```python
from build123d import *

# Parameters (mm, degrees)
SKETCH_1_W                         = 12
SKETCH_1_H                         = 8
EXTRUDE_1_DEPTH                    = 350
CUT_EXTRUDE_1_DEPTH                = 351
CHAMFER_1_SIZE                     = 0.5
PATTERN_LINEAR_1_COUNT             = 9
PATTERN_LINEAR_1_PITCH             = 40
CHAMFER_1_OF_PATTERN_LINEAR_1_SIZE = 0.5
CHAMFER_2_SIZE                     = 0.3


with BuildPart() as part:
    # Эскиз1 → Бобышка-Вытянуть1 (new body)
    with BuildSketch(Plane(origin=(0, 0, 0), x_dir=(1, 0, 0), z_dir=(0, 1, 0))):
        with Locations((6, 4)):
            Rectangle(SKETCH_1_W, SKETCH_1_H)
    extrude(amount=EXTRUDE_1_DEPTH)

    # Эскиз2 → Вырез-Вытянуть1 (cut, through all)
    with BuildSketch(Plane(origin=(0, 350, 0), x_dir=(1, 0, 0), z_dir=(0, 1, 0))):
        with BuildLine():
            Line((11, 2.25), (11, 1.75))
            Line((11, 1.75), (11.5, 1.75))
            ThreePointArc((11.5, 1.75), (11.706107374, 1.524471742), (12, 1.440983006))
            Line((12, 1.440983006), (12, 2.559016994))
            ThreePointArc((12, 2.559016994), (11.706107374, 2.475528258), (11.5, 2.25))
            Line((11.5, 2.25), (11, 2.25))
        make_face()
    cut_extrude_1 = extrude(amount=-CUT_EXTRUDE_1_DEPTH, mode=Mode.SUBTRACT)

    # Зеркальное отражение1: Вырез-Вытянуть1 across plane
    add(cut_extrude_1.mirror(Plane(origin=(6, 0, 0), x_dir=(0, 0, 1), z_dir=(1, 0, 0))), mode=Mode.SUBTRACT)

    # Эскиз4 → Вырез-Повернуть1 (revolve, cut)
    with BuildSketch(Plane(origin=(6, 0, 0), x_dir=(0, 0, -1), z_dir=(1, 0, 0))):
        Polygon((0, 339), (4.5, 339), (4.5, 337.25), (8, 337.25), (8, 335), (0, 335), align=None)
    cut_revolve_1 = revolve(axis=Axis((6, 335, -8), (0, 0, 1)), mode=Mode.SUBTRACT)

    # Фаска1
    chamfer_1_edges = [part.edges().sort_by_distance(p)[0] for p in [
        (6, 331, 0),
        (6, 332.75, -8),
    ]]
    chamfer(chamfer_1_edges, length=CHAMFER_1_SIZE)

    # Линейный массив1: Вырез-Повернуть1 ×9
    with Locations(*[(0, -i * PATTERN_LINEAR_1_PITCH, 0) for i in range(1, PATTERN_LINEAR_1_COUNT)]):
        add(cut_revolve_1, mode=Mode.SUBTRACT)

    # Фаска1 of Линейный массив1
    chamfer_1_of_pattern_linear_1_edges = [part.edges().sort_by_distance(p)[0] for p in [
        (6, 291, 0),
        (6, 292.75, -8),
        (6, 251, 0),
        (6, 252.75, -8),
        (6, 211, 0),
        (6, 212.75, -8),
        (6, 171, 0),
        (6, 172.75, -8),
        (6, 131, 0),
        (6, 132.75, -8),
        (6, 91, 0),
        (6, 92.75, -8),
        (6, 51, 0),
        (6, 52.75, -8),
        (6, 11, 0),
        (6, 12.75, -8),
    ]]
    chamfer(chamfer_1_of_pattern_linear_1_edges, length=CHAMFER_1_OF_PATTERN_LINEAR_1_SIZE)

    # Фаска2
    chamfer_2_edges = [part.edges().sort_by_distance(p)[0] for p in [
        (12, 350, -0.720491503),
        (6, 350, -8),
        (12, 0, -5.279508497),
        (12, 350, -5.279508497),
        (11.25, 0, -2.25),
        (11.706107374, 0, -2.475528258),
        (11.706107374, 0, -1.524471742),
        (11.25, 0, -1.75),
        (11, 0, -2),
        (11.25, 350, -2.25),
        (11, 350, -2),
        (11.25, 350, -1.75),
        (11.706107374, 350, -1.524471742),
        (11.706107374, 350, -2.475528258),
        (0, 0, -0.720491503),
        (0, 350, -0.720491503),
        (0, 350, -5.279508497),
        (0.75, 350, -2.25),
        (1, 350, -2),
        (0.75, 350, -1.75),
        (0.293892626, 350, -1.524471742),
        (0.293892626, 350, -2.475528258),
        (0.75, 0, -2.25),
        (6, 0, -8),
        (1, 0, -2),
        (0.75, 0, -1.75),
        (0.293892626, 0, -1.524471742),
        (0.293892626, 0, -2.475528258),
        (12, 0, -0.720491503),
        (6, 0, 0),
        (0, 0, -5.279508497),
        (6, 350, 0),
        (0, 175, -8),
        (12, 175, -8),
        (12, 175, 0),
        (0, 175, 0),
    ]]
    chamfer(chamfer_2_edges, length=CHAMFER_2_SIZE)


solid = part.part
```
Can you work these out from the model? Positions are in its coordinate system, mm. Round coordinates to 2 decimals unless told otherwise and drop trailing zeros. Order: outer loops, then holes, each group sorted by start corner. A loop starts at its lowest first (then second) coordinate and runs counter-clockwise, first axis right, second up.
(1) If we section it at B-B (x = 6): Count the separate pieces of the cut face and the enclosed holes in it, plus the area to 3 significant figures.
Results are:
separate pieces: 10
enclosed holes: 0
area: 2,330 mm2
(2) I'm going to push flat-ended pins straight in: pin 1 (0.6 mm diameter, centred on y = 93.5, z = -2, fed in from +X); pin 2 (5 mm diameter, centred on x = 6, y = 215, fed in from -Z); pin 3 (2.5 mm diameter, centred on x = 7, y = 174.5, fed in from +Z). Where does each tip first touch, or does it pass through?
Results are:
pin 1: stops at x = 11.53
pin 2: stops at z = -7.75
pin 3: stops at z = -4.5
(3) If we section it at A-A (y = 273): Please give me the cut outline in (x, z).
Results are:
outline: (0, -7.7) - (0.3, -8) - (11.7, -8) - (12, -7.7) - (12, -2.56) arc R0.56 cw to (11.5, -2.25) - (11, -2.25) - (11, -1.75) - (11.5, -1.75) arc R0.56 cw to (12, -1.44) - (12, -0.3) - (11.7, 0) - (0.3, 0) - (0, -0.3) - (0, -1.44) arc R0.56 cw to (0.5, -1.75) - (1, -1.75) - (1, -2.25) - (0.5, -2.25) arc R0.56 cw to (0, -2.56) - close
(4) If I drill on L1, parallel to Z at x = 11.25, y = 200.5; L2, parallel to X at y = 255, z = -6.55; L3, parallel to X at y = 215, z = -2.2, over which ranges is the centre line in solid material (lowest first)?
Results are:
L1: z = -8 to -2.25, -1.75 to 0
L2: x = 0 to 3.75, 8.25 to 12
L3: x = 1 to 2, 10 to 11
